```python
from build123d import *

# Parameters (mm, degrees)
CYLINDER_DEPTH      = 5
CYLINDER_DEPTH_BACK = 10
SKETCH_1_R          = 7.5
SKETCH_1_R_2        = 2
SKETCH_2_R          = 36.75
SKETCH_2_R_2        = 2.5
BASE_HORIZONT_DEPTH = 5
SKETCH_3_R          = 32.75
SKETCH_3_R_2        = 28.75
EDGE_2_DEPTH        = 15
CUTOFF_DEPTH        = 10
CUTOFF_DEPTH_BACK   = 10
SKETCH_8_W          = 61.662387238
SKETCH_8_H          = 16.75
SKETCH_12_W         = 8
SKETCH_12_H         = 4
CUT_EXTRUDE_1_DEPTH = 10
EXTRUDE_2_DEPTH     = 10
SKETCH_14_R         = 2
CUT_EXTRUDE_3_DEPTH = 10


with BuildPart() as part:
    # Эскиз1 → cylinder (new, two sides: drawn at the far end of the back side and taken through both)
    with BuildSketch(Plane(origin=(0, 0, 0), x_dir=(1, 0, 0), z_dir=(0, 1, 0)).offset(-CYLINDER_DEPTH_BACK)):
        with Locations(Location((0, 0, 0), (0, 0, 270))):
            Circle(SKETCH_1_R)
        with Locations(Location((0, 0, 0), (0, 0, 270))):
            Circle(SKETCH_1_R_2, mode=Mode.SUBTRACT)
    extrude(amount=CYLINDER_DEPTH + CYLINDER_DEPTH_BACK)

    # Эскиз2 → base horizont (add)
    with BuildSketch(Plane(origin=(0, 0, 0), x_dir=(1, 0, 0), z_dir=(0, 1, 0))):
        with Locations(Location((0, 0, 0), (0, 0, 270))):
            Circle(SKETCH_2_R)
        Circle(SKETCH_2_R_2, mode=Mode.SUBTRACT)
    extrude(amount=BASE_HORIZONT_DEPTH)

    # Эскиз3 → edge 2 (add)
    with BuildSketch(Plane(origin=(0, 5, 0), x_dir=(1, 0, 0), z_dir=(0, 1, 0))):
        with Locations(Location((0, 0, 0), (0, 0, 270))):
            Circle(SKETCH_3_R)
        with Locations(Location((0, 0, 0), (0, 0, 270))):
            Circle(SKETCH_3_R_2, mode=Mode.SUBTRACT)
    extrude(amount=-EDGE_2_DEPTH)

    # Эскиз8 → cutoff (cut, two sides: drawn at the far end of the back side and taken through both)
    with BuildSketch(Plane(origin=(0, 0, 0), x_dir=(1, 0, 0), z_dir=(0, 1, 0)).offset(-CUTOFF_DEPTH_BACK)):
        with Locations((0, 28.375)):
            Rectangle(SKETCH_8_W, SKETCH_8_H)
    extrude(amount=CUTOFF_DEPTH + CUTOFF_DEPTH_BACK, mode=Mode.SUBTRACT)

    # Эскиз12 → Вытянуть1 (cut)
    with BuildSketch(Plane.XZ.offset(10)):
        with Locations((-24.575557737, -18)):
            Rectangle(SKETCH_12_W, SKETCH_12_H)
        with Locations((24.575557737, -18)):
            Rectangle(SKETCH_12_W, SKETCH_12_H)
    extrude(amount=-CUT_EXTRUDE_1_DEPTH, mode=Mode.SUBTRACT)

    # Эскиз13 → Вытянуть2 (add)
    with BuildSketch(Plane.XZ):
        with BuildLine():
            Line((-30.831193619, 20), (-25.933809978, 20))
            ThreePointArc((-25.933809978, 20), (-27.636674985, 17.572043016), (-29.112926682, 15))
            Line((-29.112926682, 15), (-33.54940387, 15))
            ThreePointArc((-33.54940387, 15), (-32.287231737, 17.552696851), (-30.831193619, 20))
        make_face()
        with BuildLine():
            Line((33.54940387, 15), (29.112926682, 15))
            ThreePointArc((29.112926682, 15), (27.636674985, 17.572043016), (25.933809978, 20))
            Line((25.933809978, 20), (30.831193619, 20))
            ThreePointArc((30.831193619, 20), (32.287231737, 17.552696851), (33.54940387, 15))
        make_face()
    extrude(amount=EXTRUDE_2_DEPTH)

    # Эскиз14 → Вытянуть3 (cut)
    with BuildSketch(Plane(origin=(0, 5, 0), x_dir=(1, 0, 0), z_dir=(0, 1, 0))):
        with Locations(Location((14, -14, 0), (0, 0, 270))):
            Circle(SKETCH_14_R)
        with Locations(Location((-14, -14, 0), (0, 0, 270))):
            Circle(SKETCH_14_R)
        with Locations(Location((-14, 14, 0), (0, 0, 270))):
            Circle(SKETCH_14_R)
        with Locations(Location((14, 14, 0), (0, 0, 270))):
            Circle(SKETCH_14_R)
    extrude(amount=-CUT_EXTRUDE_3_DEPTH, mode=Mode.SUBTRACT)


solid = part.part
```
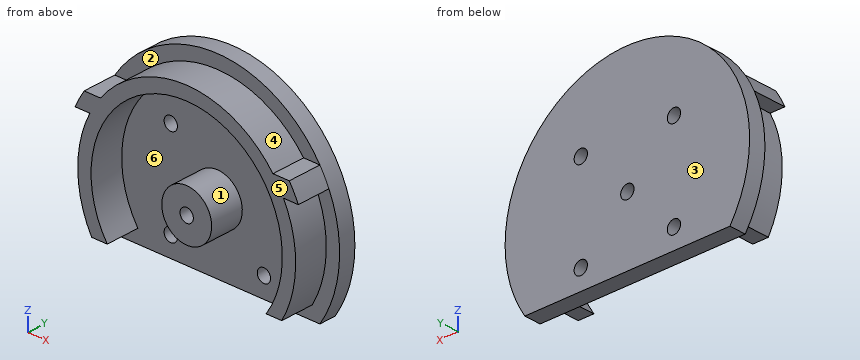
The model under review builds one solid part; all positions refer to its coordinate system, in mm. Face numbers are marked on the shaded views. A direction names the side the tool comes from. Coordinates: 2 decimals unless noted, no trailing zeros. Write each loop counter-clockwise with the first axis right and the second up, starting at its lowest first coordinate (ties: lowest second). Pieces come first, ordered by that corner, then holes. Notation, with made-up numbers: (82, -0.75) - (113, -0.75) arc R16 ccw to (113, 6.25) - close; hole circle Ø5 at (-39, 63.5). An arc over 180 degrees is marked (long way). Answer in a Markdown table with one row per item. Add a question column.
Q1. To check wall thickness, follow line 1 along X through (y, z) = (-4.25, 0); line 2 along Y through (x, z) = (9, -8.5); line 3 along X through (y, z) = (1.85, 14). State the ranges of each line that lie inside material, in increasing order. Write a range as from..to.
Q2. Consider section B-B on z = 0. Give the boundary of the cut face in (x, y), then the cut area to 4 significant figures.
Q3. Draft analysis for pull direction Z (two halves, no side actions). For the marked faces 4, 5 and 6, state which applies: +Z half, -Z half, draft (parallel to the pull), parting line (faces both ways), or undercut.
Q4. Consider section A-A on y = -1. Give the boundary of the cut face in (x, z), then the cut area to 3 significant figures.
Q5. Consider section D-D on x = -9. Give the boundary of the cut face in (y, z) (3 decimals).
Q6. Clearance check with flat-ended pins moving along their axes: pin 1 (5 mm diameter, centred on x = 31.5, y = -4, fed in from -Z); pin 2 (3.5 mm diameter, centred on x = -30.5, y = -5, fed in from -Z); pin 3 (4 mm diameter, centred on y = -4, z = 15, fed in from -X). State where each tip first meets the part, or that it passes through.
Q7. Consider section C-C on z = -14. Give the boundary of the cut face in (x, y).
Q8. For the marked faces 1, 2 and 3, list the 3-axis set-ups (+Z, -Z, +X, -X, +Y, -Y) from which the entire face can be reached by the end or side of a thin tool; tool diameter is ignored.
Answers below:
| question | item | result |
|---|---|---|
| 1 | line 1 | -32.75..-28.75, -7.5..-2, 2..7.5, 28.75..32.75 |
| 1 | line 2 | 0..5 |
| 1 | line 3 | -33.98..-16, -12..12, 16..33.98 |
| 2 | outline | (-36.75, 0) - (-32.75, 0) - (-32.75, -10) - (-28.75, -10) - (-28.75, 0) - (-7.5, 0) - (-7.5, -10) - (-2, -10) - (-2, 5) - (-36.75, 5) - close; (2, -10) - (7.5, -10) - (7.5, 0) - (28.75, 0) - (28.75, -10) - (32.75, -10) - (32.75, 0) - (36.75, 0) - (36.75, 5) - (2, 5) - close |
| 2 | area | 537.5 mm² |
| 3 | face 4 | +Z half |
| 3 | face 5 | draft |
| 3 | face 6 | undercut |
| 4 | outline | (-33.55, 15) - (-29.11, 15) arc R32.75 ccw to (-28.58, -16) - (-23.89, -16) arc R28.75 cw (long way) to (23.89, -16) - (28.58, -16) arc R32.75 ccw to (29.11, 15) - (33.55, 15) arc R36.75 ccw to (30.83, 20) - (25.93, 20) arc R32.75 ccw to (-25.93, 20) - (-30.83, 20) arc R36.75 ccw to start; circle Ø15 at (0, 0); hole circle Ø4 at (0, 0) |
| 4 | area | 732 mm² |
| 5 | outline | (-10, 27.305) - (0, 27.305) - (0, -20) - (5, -20) - (5, 35.631) - (0, 35.631) - (0, 31.489) - (-10, 31.489) - close |
| 6 | pin 1 | z = -15.22 |
| 6 | pin 2 | z = -15.68 |
| 6 | pin 3 | x = -33.55 |
| 7 | outline | (-33.98, 0) - (-29.61, 0) - (-29.61, -10) - (-25.11, -10) - (-25.11, 0) - (-16, 0) - (-16, 5) - (-33.98, 5) - close; (-12, 0) - (12, 0) - (12, 5) - (-12, 5) - close; (16, 0) - (25.11, 0) - (25.11, -10) - (29.61, -10) - (29.61, 0) - (33.98, 0) - (33.98, 5) - (16, 5) - close |
| 8 | face 1 | -Y |
| 8 | face 2 | +Z, -Y |
| 8 | face 3 | +Z, -Z, +X, -X, +Y |
